The listing builds one solid part. Answer for the finished solid, in the listing's coordinates (mm). A direction names the side the tool comes from. Give positions to 0.01 mm unless a question says otherwise; leave off trailing zeros. Order: outer loops, then holes, each group sorted by start corner. A loop starts at its lowest first (then second) coordinate and runs counter-clockwise, first axis right, second up. Notation, with made-up numbers: (-26.5, -25) - (3.5, -25) arc R11 cw to (3.5, -18) - close; hole circle Ø11 at (43, 87.25). An arc over 180 degrees is marked (long way). Answer as a JSON object with one key per item and string values. Group by question number.
Q1. The mould has two halves that part along Z. Classify faces 5 (the face through (-5, 1, 16)), 6 (the face through (8, 9, 6)), 7 (the face through (5, 11.487, 15)): released by +Z, released by -Z, zero draft, split by the parting line, or undercut.
Q2. A cutting plane is placed at D-D, the plane x = -6.5. Give the vertices of the cut face in (y, z).
Q3. A cutting plane is placed at B-B, the plane x = 0. Give the vertices of the cut face in (y, z).
Q4. For faces 1 (the face through (-7.622, 11.535, 8.322)), 2 (the face through (5.4, -10.7, 15.5)), 3 (the face through (2.699, 0.2, 15.2)), 4 (the face through (8.096, 0.2, 15.2)), determine the directions among +Z, -Z, +X, -X, +Y, -Y from which every point of the face is accessible in a straight line to the end or side of a thin tool.
Q5. Consider line 1 (Y direction, x = 0, z = 6.75); line 2 (X direction, y = 6.5, z = 15.25); line 3 (Z direction, x = 6, y = 11). Determine where each line is inside the solid, lowest interval first.
Q6. A cutting plane is placed at C-C, the plane z = 14.5. Give the vertices of the cut face in (x, y).
Q7. Given pin 1 (2 mm diameter, centred on x = 6, z = 15, fed in from +Y); pin 2 (1.1 mm diameter, centred on x = -7.5, z = 6.5, fed in from +Y); pin 3 (1.5 mm diameter, centred on x = 0, y = 0, fed in from -Z), each flat-ended and moving along its own axis, determine where each tip first touches the part or whether it passes through.
Q8. A cutting plane is placed at A-A, the plane y = 0. Give the vertices of the cut face in (x, z).
from build123d import *

# Parameters (mm, degrees)
SKETCH1_W           = 20
SKETCH1_H           = 28
BOSS_EXTRUDE1_DEPTH = 15
CUT_EXTRUDE1_DEPTH  = 21
CUT_EXTRUDE2_DEPTH  = 5
SKETCH4_W           = 5.397016415
SKETCH4_H           = 22.187734152
BOSS_EXTRUDE2_DEPTH = 1
SKETCH5_R           = 1.25
CUT_EXTRUDE3_DEPTH  = 16


with BuildPart() as part:
    # Sketch1 → Boss-Extrude1 (new body)
    with BuildSketch(Plane.XY):
        Rectangle(SKETCH1_W, SKETCH1_H)
    extrude(amount=BOSS_EXTRUDE1_DEPTH)

    # Sketch2 → Cut-Extrude1 (cut, through all)
    with BuildSketch(Plane(origin=(10, 0, 0), x_dir=(0, 0, -1), z_dir=(1, 0, 0))):
        Polygon((-11.5, 14), (-15, 14), (-15, 6), align=None)
    extrude(amount=-CUT_EXTRUDE1_DEPTH, mode=Mode.SUBTRACT)

    # Sketch3 → Cut-Extrude2 (cut)
    with BuildSketch(Plane(origin=(0, 14, 0), x_dir=(1, 0, 0), z_dir=(0, 1, 0))):
        with BuildLine():
            Line((4.654488589, -4.572843843), (4.654488589, -6.572843843))
            ThreePointArc((4.654488589, -6.572843843), (2.904488589, -8.322843843), (1.154488589, -6.572843843))
            Line((1.154488589, -6.572843843), (1.154488589, -4.572843843))
            ThreePointArc((1.154488589, -4.572843843), (2.904488589, -2.822843843), (4.654488589, -4.572843843))
        make_face()
        with BuildLine():
            Line((9.333625698, -4.572843843), (9.333625698, -6.572843843))
            ThreePointArc((9.333625698, -6.572843843), (7.583625698, -8.322843843), (5.833625698, -6.572843843))
            Line((5.833625698, -6.572843843), (5.833625698, -4.572843843))
            ThreePointArc((5.833625698, -4.572843843), (7.583625698, -2.822843843), (9.333625698, -4.572843843))
        make_face()
    cut_extrude2 = extrude(amount=-CUT_EXTRUDE2_DEPTH, mode=Mode.SUBTRACT)

    # Sketch4 → Boss-Extrude2 (add, symmetric)
    with BuildSketch(Plane.XY.offset(15)):
        with Locations((5.397016416, 0.393532447)):
            Rectangle(SKETCH4_W, SKETCH4_H)
    boss_extrude2 = extrude(amount=BOSS_EXTRUDE2_DEPTH, both=True)

    # Mirror1: Cut-Extrude2, Boss-Extrude2 across plane
    add(cut_extrude2.mirror(Plane(origin=(0, 0, 0), x_dir=(0, 0, 1), z_dir=(1, 0, 0))), mode=Mode.SUBTRACT)
    add(boss_extrude2.mirror(Plane(origin=(0, 0, 0), x_dir=(0, 0, 1), z_dir=(1, 0, 0))))

    # Sketch5 → Cut-Extrude3 (cut, through all)
    with BuildSketch(Plane.XY.offset(15)):
        Circle(SKETCH5_R)
    extrude(amount=-CUT_EXTRUDE3_DEPTH, mode=Mode.SUBTRACT)


solid = part.part
Reply:
{
 "1": {"face 5": "released by +Z", "face 6": "undercut", "face 7": "zero draft"},
 "2": {"outline": "(-14, 0) - (14, 0) - (14, 3.2) - (9, 3.2) - (9, 7.95) - (14, 7.95) - (14, 11.5) - (8.29, 14) - (11.49, 14) - (11.49, 16) - (-10.7, 16) - (-10.7, 15) - (-14, 15) - close"},
 "3": {"outline": "(-14, 0) - (-1.25, 0) - (-1.25, 15) - (-14, 15) - close; (1.25, 0) - (14, 0) - (14, 11.5) - (6, 15) - (1.25, 15) - close"},
 "4": {"face 1": "+Y", "face 2": "+Z, +X, -X, -Y", "face 3": "+Z, +Y", "face 4": "+Z, +X, +Y"},
 "5": {"line 1": "y = -14 to -1.25, 1.25 to 14", "line 2": "x = -8.1 to -2.7, 2.7 to 8.1", "line 3": "z = 0 to 3.83, 7.32 to 12.81, 14 to 16"},
 "6": {"outline": "(-10, -14) - (10, -14) - (10, 7.14) - (8.1, 7.14) - (8.1, 11.49) - (2.7, 11.49) - (2.7, 7.14) - (-2.7, 7.14) - (-2.7, 11.49) - (-8.1, 11.49) - (-8.1, 7.14) - (-10, 7.14) - close; hole circle Ø2.5 at (0, 0)"},
 "7": {"pin 1": "stops at y = 11.49", "pin 2": "stops at y = 9", "pin 3": "passes through"},
 "8": {"outline": "(-10, 0) - (-1.25, 0) - (-1.25, 15) - (-2.7, 15) - (-2.7, 16) - (-8.1, 16) - (-8.1, 15) - (-10, 15) - close; (1.25, 0) - (10, 0) - (10, 15) - (8.1, 15) - (8.1, 16) - (2.7, 16) - (2.7, 15) - (1.25, 15) - close"}
}
